The model under review builds one solid part; all positions refer to its coordinate system, in mm. Face numbers are marked on the shaded views. A direction names the side the tool comes from. Coordinates: 2 decimals unless noted, no trailing zeros. Order: outer loops, then holes, each group sorted by start corner. A loop starts at its lowest first (then second) coordinate and runs counter-clockwise, first axis right, second up. Notation, with made-up numbers: M 45,-37.5 L 92,-37.5 A23 ccw 92,-9.5 Z; hole C 44.5,-28.5 d2. An arc over 180 degrees is marked long. One line per item, written item: value.
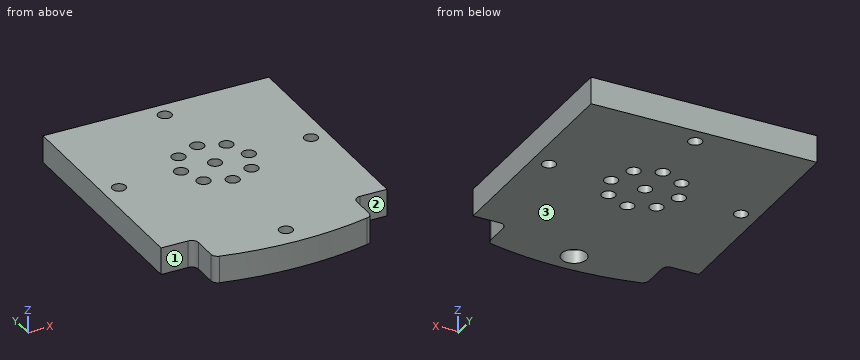
```python
from build123d import *

# Parameters (mm, degrees)
SKETCH_1_R          = 3
EXTRUDE_1_DEPTH     = 12
SKETCH_3_R          = 5.5
CUT_EXTRUDE_2_DEPTH = 6


with BuildPart() as part:
    # 草图1 → 凸台-拉伸1 (new body)
    with BuildSketch(Plane.XY):
        with BuildLine():
            Line((-35, -53), (-35, -63.474736452))
            ThreePointArc((-35, -63.474736452), (-34.340852801, -65.351011529), (-32.653061224, -66.402792298))
            ThreePointArc((-32.653061224, -66.402792298), (0, -70), (32.653061224, -66.402792298))
            ThreePointArc((32.653061224, -66.402792298), (34.340852801, -65.351011529), (35, -63.474736452))
            Line((35, -63.474736452), (35, -53))
            ThreePointArc((35, -53), (35.878679656, -50.878679656), (38, -50))
            Line((38, -50), (50, -50))
            Line((50, -50), (50, 50))
            Line((50, 50), (0, 50))
            Line((0, 50), (-50, 50))
            Line((-50, 50), (-50, -50))
            Line((-50, -50), (-38, -50))
            ThreePointArc((-38, -50), (-35.878679656, -50.878679656), (-35, -53))
        make_face()
        with Locations((-42.5, 0)):
            Circle(SKETCH_1_R, mode=Mode.SUBTRACT)
        with Locations((42.5, 0)):
            Circle(SKETCH_1_R, mode=Mode.SUBTRACT)
        with Locations((0, -60)):
            Circle(SKETCH_1_R, mode=Mode.SUBTRACT)
        Circle(SKETCH_1_R, mode=Mode.SUBTRACT)
        with Locations((0, 42.5)):
            Circle(SKETCH_1_R, mode=Mode.SUBTRACT)
        with Locations((15, 0)):
            Circle(SKETCH_1_R, mode=Mode.SUBTRACT)
        with Locations((10.606601718, -10.606601718)):
            Circle(SKETCH_1_R, mode=Mode.SUBTRACT)
        with Locations((0, -15)):
            Circle(SKETCH_1_R, mode=Mode.SUBTRACT)
        with Locations((-10.606601718, -10.606601718)):
            Circle(SKETCH_1_R, mode=Mode.SUBTRACT)
        with Locations((-15, 0)):
            Circle(SKETCH_1_R, mode=Mode.SUBTRACT)
        with Locations((-10.606601718, 10.606601718)):
            Circle(SKETCH_1_R, mode=Mode.SUBTRACT)
        with Locations((0, 15)):
            Circle(SKETCH_1_R, mode=Mode.SUBTRACT)
        with Locations((10.606601718, 10.606601718)):
            Circle(SKETCH_1_R, mode=Mode.SUBTRACT)
    extrude(amount=EXTRUDE_1_DEPTH)

    # 草图3 → 切除-拉伸2 (cut)
    with BuildSketch(Plane(origin=(0, 0, 0), x_dir=(-1, 0, 0), z_dir=(0, 0, -1))):
        with Locations((0, -60)):
            Circle(SKETCH_3_R)
    extrude(amount=-CUT_EXTRUDE_2_DEPTH, mode=Mode.SUBTRACT)


solid = part.part
```
(1) Tool access review of the marked faces 1, 2 and 3: name each direction out of +Z, -Z, +X, -X, +Y, -Y from which nothing blocks a thin tool from reaching the whole face with its end or side.
Geometry results:
face 1: +Z, -Z, -X, -Y
face 2: +Z, -Z, +X, -Y
face 3: -Z, +X, -X, +Y, -Y
(2) We need section B-B, the plane x = 0. State the section outline as (y, z) points.
Geometry results:
outline: M -70,0 L -65.5,0 L -65.5,6 L -63,6 L -63,12 L -70,12 Z; M -57,6 L -54.5,6 L -54.5,0 L -18,0 L -18,12 L -57,12 Z; M -12,0 L -3,0 L -3,12 L -12,12 Z; M 3,0 L 12,0 L 12,12 L 3,12 Z; M 18,0 L 39.5,0 L 39.5,12 L 18,12 Z; M 45.5,0 L 50,0 L 50,12 L 45.5,12 Z
(3) For L1, parallel to Y at x = 8, z = 8.75; L2, parallel to Y at x = -11.5, z = 8; L3, parallel to X at y = -53, z = 8, list the stretches that pass through material, from the lowest coordinate up.
Geometry results:
L1: y = -69.79 to -12.09, -9.12 to 9.12, 12.09 to 50
L2: y = -69.56 to -13.47, -7.74 to 7.74, 13.47 to 50
L3: x = -35 to 35
(4) We need section D-D, the plane z = 4.25. Count the separate pieces of the cut face and the enclosed holes in it, plus the area to 3 significant figures.
Geometry results:
separate pieces: 1
enclosed holes: 13
area: 10,900 mm2
(5) Insertion check: pin 1 Ø3 at (y, z) = (-59, 5) entering from +X; pin 2 Ø8 at (x, y) = (0, -60) entering from -Z. Each pin has a flat end and moves straight along its axis. Give the tip position at first contact, or say it passes through.
Geometry results:
pin 1: stops at x = 35
pin 2: stops at z = 6
(6) We need section C-C, the plane y = 0. State the section outline as (x, z) points, plus the area to 3 significant figures.
Geometry results:
outline: M -50,0 L -45.5,0 L -45.5,12 L -50,12 Z; M -39.5,0 L -18,0 L -18,12 L -39.5,12 Z; M -12,0 L -3,0 L -3,12 L -12,12 Z; M 3,0 L 12,0 L 12,12 L 3,12 Z; M 18,0 L 39.5,0 L 39.5,12 L 18,12 Z; M 45.5,0 L 50,0 L 50,12 L 45.5,12 Z
area: 840 mm2
(7) We need section A-A, the plane y = 15. State the section outline as (x, z) points, plus the area to 3 significant figures.
Geometry results:
outline: M -50,0 L -3,0 L -3,12 L -50,12 Z; M 3,0 L 50,0 L 50,12 L 3,12 Z
area: 1,130 mm2
